Study the drawing (mm; zero at the part's minimum x, y, z) and answer. Coordinates: 2 decimals unless noted, no trailing zeros. Order: outer loops, then holes, each group sorted by start corner. A loop starts at its lowest first (then second) coordinate and runs counter-clockwise, first axis right, second up.
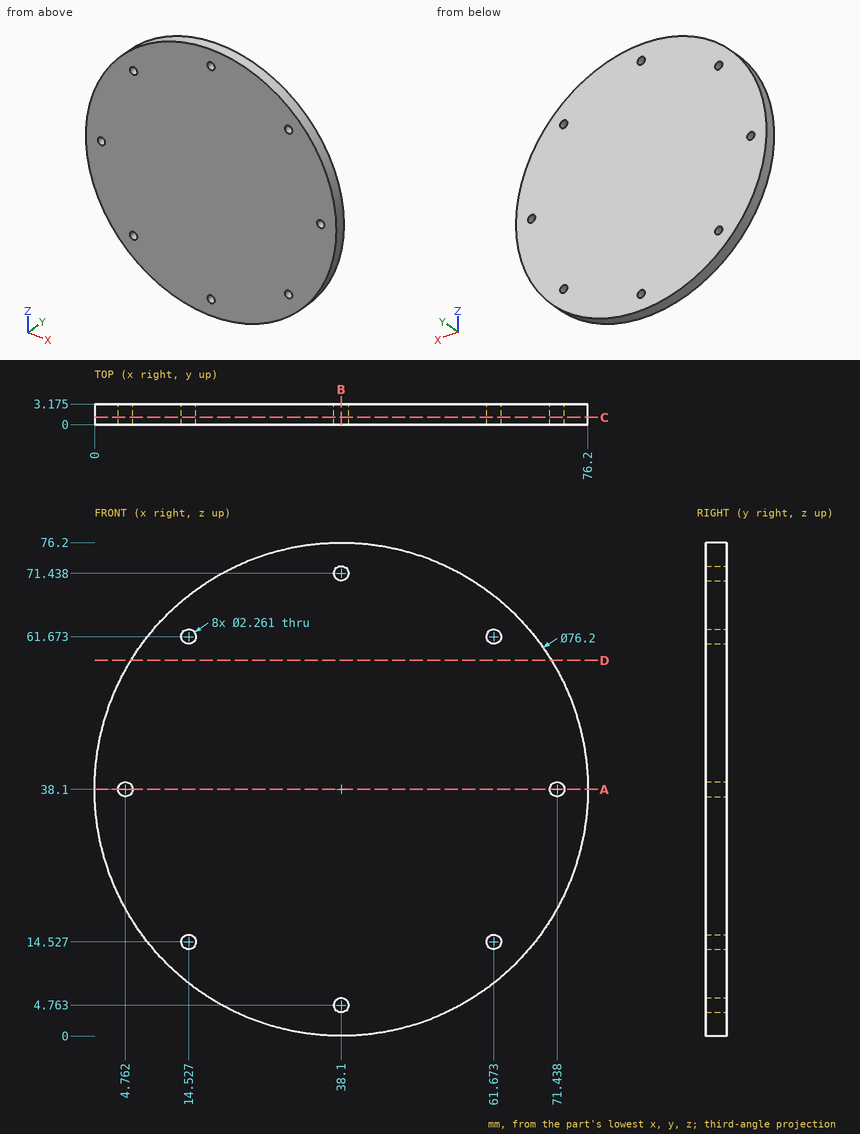
(1) Find section C-C on y = 1.1. Count the separate pieces of the cut face and the enclosed holes in it, then the cut area to 3 significant figures.
(2) Find the intervals of material crossed by probe 1 along X at (y, z) = (2.3, 38.1); probe 2 along Z at (x, y) = (38, 0.3); probe 3 along Z at (x, y) = (14, 1.6) (1 decimal), in increasing order.
(3) Find section D-D on z = 58. Determine the outline of the cut face in (x, y) (1 decimal).
(4) Find section A-A on z = 38.1. Determine the outline of the cut face in (x, y) (1 decimal).
(5) Find section B-B on x = 38.1. Determine the outline of the cut face in (y, z) (1 decimal).
(6) Given pin 1 Ø1.8 at (x, z) = (61.67, 14.53) entering from -Y; pin 2 Ø1 at (x, y) = (34, 2) entering from +Z, each flat-ended and moving along its own axis, determine where each tip first touches the part or whether it passes through.
Resolved:
1. separate pieces: 1
1. enclosed holes: 8
1. area: 4,530 mm2
2. probe 1: x = 0 to 3.63, 5.89 to 70.31, 72.57 to 76.2
2. probe 2: z = 0 to 3.64, 5.89 to 70.31, 72.56 to 76.2
2. probe 3: z = 8.6 to 13.5, 15.5 to 60.7, 62.7 to 67.6
3. outline: (5.6, 0) - (70.6, 0) - (70.6, 3.2) - (5.6, 3.2) - close
4. outline: (0, 0) - (3.6, 0) - (3.6, 3.2) - (0, 3.2) - close; (5.9, 0) - (70.3, 0) - (70.3, 3.2) - (5.9, 3.2) - close; (72.6, 0) - (76.2, 0) - (76.2, 3.2) - (72.6, 3.2) - close
5. outline: (0, 0) - (3.2, 0) - (3.2, 3.6) - (0, 3.6) - close; (0, 5.9) - (3.2, 5.9) - (3.2, 70.3) - (0, 70.3) - close; (0, 72.6) - (3.2, 72.6) - (3.2, 76.2) - (0, 76.2) - close
6. pin 1: passes through
6. pin 2: stops at z = 76.03
